Model file for the job. Use its own axes, mm. Face numbers are marked on the shaded views. Round coordinates to 2 decimals unless told otherwise and drop trailing zeros. Loops run counter-clockwise (first coordinate to the right, second up) from the corner with the lowest first, then second, coordinate; pieces in that order, holes last. Notation, with made-up numbers: M -2,-5.75 L 10,-5.75 A20 cw 10,17.25 Z; hole C -15.5,58.25 d5. An arc over 180 degrees is marked long. Answer in a Markdown table with one row per item.
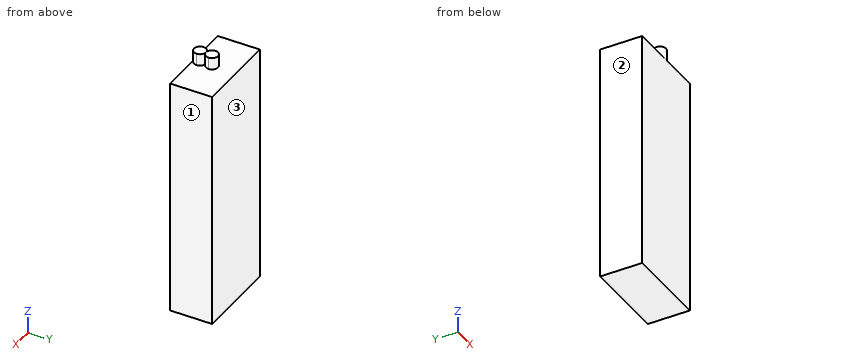
Autodesk Inventor part; units mm, degrees
ref_plane "YZ Plane" through (0, 0, 0) normal (1, 0, 0) x (0, 1, 0)
ref_plane "XZ Plane" through (0, 0, 0) normal (0, 1, 0) x (-1, 0, 0)
ref_plane "XY Plane" through (0, 0, 0) normal (0, 0, 1) x (1, 0, 0)
sketch "Sketch1" plane through (0, 0, 0) normal (0, 1, 0) x (-1, 0, 0)
  line L0 (0, 0) -> (70, 0)
  line L1 (70, 0) -> (70, -200)
  line L2 (70, -200) -> (0, -200)
  line L3 (0, -200) -> (0, 0)
  dimension "d0" = 70
  dimension "d1" = 200
extrude "Extrusion1" add sketch "Sketch1" along normal blind 35
sketch "Sketch2" plane through (-70, 0, 0) normal (0, 0, 1) x (1, 0, 0)
  point P0 (70, 0)
sketch "Sketch3" plane through (-70, 0, 0) normal (0, 0, 1) x (1, 0, 0)
  circle A0 centre (35, 5) radius 5
  circle A1 centre (35, 15) radius 5
  line L0 (70, 0) -> (70, 35)
  line L1 (0, 0) -> (70, 0)
  point P0 (70, 17.5)
  dimension "d4" = 10
  dimension "d5" = 10
  dimension "d6" = 35
  dimension "d7" = 35
  dimension "d8" = 10
  dimension "d9" = 5
extrude "Extrusion2" add sketch "Sketch3" along normal blind 10 contours A0
sketch "Sketch4" plane through (-70, 35, 0) normal (0, 0, 1) x (1, 0, 0)
  circle A0 centre (35, -20) radius 5
  line L0 (35, -35) -> (70, -35)
  line L1 (70, -35) -> (70, 0)
  dimension "d12" = 10
  dimension "d13" = 15
  dimension "d14" = 35
extrude "Extrusion3" add sketch "Sketch4" along normal blind 10
properties part number "water tank mm"
1. Saw through at C-C (y = 28). Write the cut outline in (x, z), and give its area (3 significant figures).
Verdict:
| item | result |
|---|---|
| outline | M -70,-200 L 0,-200 L 0,0 L -70,0 Z |
| area | 14,000 mm² |
2. Saw through at A-A (y = 8). Write the cut outline in (x, z).
Verdict:
| item | result |
|---|---|
| outline | M -70,-200 L 0,-200 L 0,0 L -31,0 L -31,10 L -39,10 L -39,0 L -70,0 Z |
3. Wall check: probe 1 along Z at (x, y) = (-45, 20). Give the ranges that are in metal, low to high.
Verdict:
| item | result |
|---|---|
| probe 1 | z = -200 to 0 |
4. Saw through at B-B (x = -61). Write the cut outline in (y, z), and give its area (3 significant figures).
Verdict:
| item | result |
|---|---|
| outline | M 0,-200 L 35,-200 L 35,0 L 0,0 Z |
| area | 7,000 mm² |
5. Mould opens along X. For the marked faces 1, 2 and 3 say: +X half, -X half, draft (parallel to the pull), parting line (faces both ways), or undercut.
Verdict:
| item | result |
|---|---|
| face 1 | +X half |
| face 2 | -X half |
| face 3 | draft |
6. Pin check, flat tip, straight feed: pin 1 (1.5 mm diameter, centred on x = -13, y = 17, fed in from +Z). Stop position of the tip, or through.
Verdict:
| item | result |
|---|---|
| pin 1 | stops at z = 0 |
